```python
from build123d import *

# Parameters (mm, degrees)
F0_W      = 52.5309846
F0_H      = 44.9404867
F0_R      = 1.5
F0_R_2    = 11.2530001
F1_DEPTH  = 5
F2_W      = 3.175
F2_H      = 44.9404867
F3_DEPTH  = 41.774999
F4_W      = 7.9375
F4_H      = 3.175
F5_DEPTH  = 46.774999
F6_R      = 3.96875
F7_R      = 2.2479
F8_DEPTH  = 3.175
F10_DEPTH = 52.5309846
F12_DEPTH = 19.2659
F14_DEPTH = 10.7654979
F15_R     = 7.9375
F16_DEPTH = 25.4
F17_DEPTH = 30.4370867
F18_R     = 3.175
F19_DEPTH = 19.2659
F21_DEPTH = 133
F22_R     = 7.2517
F23_R     = 1.5875


# Not quite as in the source:
# - an extrude ends at something that could not be found from the text; its depth is read off the source's solid
# - a feature names something its author has since deleted; it is built from what else it names


with BuildPart() as f1:
    # F0 (on Top) → F1 (new body)
    with BuildSketch(Plane.XY):
        with Locations((26.2654923, -22.47024335)):
            Rectangle(F0_W, F0_H)
        with Locations((10.7654979, -38.5904867)):
            Circle(F0_R, mode=Mode.SUBTRACT)
        with Locations((26.2654923, -23.0904923)):
            Circle(F0_R_2, mode=Mode.SUBTRACT)
        with Locations((41.7654867, -38.5904867)):
            Circle(F0_R, mode=Mode.SUBTRACT)
        with Locations((10.7654979, -7.5904979)):
            Circle(F0_R, mode=Mode.SUBTRACT)
        with Locations((41.7654867, -7.5904979)):
            Circle(F0_R, mode=Mode.SUBTRACT)
    extrude(amount=F1_DEPTH)

    # F2 (on face) → F3 (join)
    with BuildSketch(Plane(origin=(0, 0, 0), x_dir=(1, 0, 0), z_dir=(0, 0, -1))):
        with Locations((1.5875, 22.47024335)):
            Rectangle(F2_W, F2_H)
        with Locations((50.9434846, 22.47024335)):
            Rectangle(F2_W, F2_H)
    extrude(amount=F3_DEPTH)

    # F4 (on face) → F5 (join, through all)
    with BuildSketch(Plane(origin=(0, 0, -41.774999), x_dir=(1, 0, 0), z_dir=(0, 0, -1))):
        with Locations((-3.96875, 1.5875)):
            Rectangle(F4_W, F4_H)
        with Locations((56.4997346, 1.5875)):
            Rectangle(F4_W, F4_H)
    extrude(amount=-F5_DEPTH)

    # F6
    f6_edges = [f1.edges().sort_by_distance(p)[0] for p in [
        (60.468485, -1.5875, -41.774999),
        (60.468485, -1.5875, 5),
        (-7.9375, -1.5875, 5),
        (-7.9375, -1.5875, -41.774999),
    ]]
    fillet(f6_edges, radius=F6_R)

    # F7 (on face) → F8 (cut, through all)
    with BuildSketch(Plane(origin=(0, 0, 0), x_dir=(-1, 0, 0), z_dir=(0, 1, 0))):
        with Locations((3.96875, -37.806249)):
            Circle(F7_R)
        with Locations((3.96875, 1.03125)):
            Circle(F7_R)
        with Locations((-56.4997346, 1.03125)):
            Circle(F7_R)
        with Locations((-56.4997346, -37.806249)):
            Circle(F7_R)
    extrude(amount=-F8_DEPTH, mode=Mode.SUBTRACT)

    # F9 (on face) → F10 (cut, through all)
    with BuildSketch(Plane.YZ.offset(52.5309846)):
        Polygon((-44.9404867, -3.175), (-44.9404867, -41.774999), (-6.35, -41.774999), align=None)
    extrude(amount=-F10_DEPTH, mode=Mode.SUBTRACT)

    # F11 (on face) → F12 (join)
    with BuildSketch(Plane.XY.offset(5)):
        with BuildLine():
            Line((41.7654867, -44.9404867), (52.5309846, -44.9404867))
            Line((52.5309846, -44.9404867), (52.5309846, -30.4370867))
            Line((52.5309846, -30.4370867), (41.7654867, -30.4370867))
            Line((41.7654867, -30.4370867), (41.7654867, -35.4154867))
            ThreePointArc((41.7654867, -35.4154867), (44.9404867, -38.5904867), (41.7654867, -41.7654867))
            Line((41.7654867, -41.7654867), (41.7654867, -44.9404867))
        make_face()
        with BuildLine():
            Line((52.5309846, -20.7092423), (52.5309846, -12.7717423))
            Line((52.5309846, -12.7717423), (30.7547472146, -12.7717423))
            ThreePointArc((30.7547472146, -12.7717423), (34.966988133, -15.9550889113), (37.2636584966, -20.7092423))
            Line((37.2636584966, -20.7092423), (52.5309846, -20.7092423))
        make_face()
    extrude(amount=F12_DEPTH)

    # F13 (on face) → F14 (cut, through all)
    with BuildSketch(Plane.YZ.offset(52.5309846)):
        with BuildLine():
            Line((-40.0700367, 17.0142), (-37.6887867, 17.0142))
            Line((-37.6887867, 17.0142), (-37.6887867, 14.63295))
            ThreePointArc((-37.6887867, 14.63295), (-36.0049886773, 15.3304019773), (-35.3075367, 17.0142))
            ThreePointArc((-35.3075367, 17.0142), (-37.6887867, 19.39545), (-40.0700367, 17.0142))
        make_face()
        with BuildLine():
            Line((-37.6887867, 14.63295), (-37.6887867, 17.0142))
            Line((-37.6887867, 17.0142), (-40.0700367, 17.0142))
            ThreePointArc((-40.0700367, 17.0142), (-39.3725847227, 15.3304019773), (-37.6887867, 14.63295))
        make_face()
    extrude(amount=-F14_DEPTH, mode=Mode.SUBTRACT)

    # F15 (on face) → F16 (cut)
    with BuildSketch(Plane.XY.offset(5)):
        with Locations((26.2654923, -10.3904923)):
            Circle(F15_R)
    extrude(amount=F16_DEPTH, mode=Mode.SUBTRACT)

    # F17 (add, through all): a face of the model
    f17_faces = [f1.faces().sort_by_distance(p)[0] for p in [
        (47.14823565, -30.4370867, 14.63295),
    ]]
    extrude(f17_faces, amount=F17_DEPTH)

    # F18 (on face) → F19 (cut, through all)
    with BuildSketch(Plane.XY.offset(5)):
        with Locations((41.7654867, -7.5904979)):
            Circle(F18_R)
    extrude(amount=F19_DEPTH, mode=Mode.SUBTRACT)

    # F20 (on face) → F21 (cut, through all)
    with BuildSketch(Plane.YZ.offset(52.5309846)):
        with BuildLine():
            ThreePointArc((-16.7404923, 19.0142), (-18.1547058624, 18.4284135624), (-18.7404923, 17.0142))
            Line((-18.7404923, 17.0142), (-16.7404923, 17.0142))
            Line((-16.7404923, 17.0142), (-16.7404923, 19.0142))
        make_face()
        with BuildLine():
            Line((-16.7404923, 17.0142), (-18.7404923, 17.0142))
            ThreePointArc((-18.7404923, 17.0142), (-16.7404923, 15.0142), (-14.7404923, 17.0142))
            ThreePointArc((-14.7404923, 17.0142), (-15.3262787376, 18.4284135624), (-16.7404923, 19.0142))
            Line((-16.7404923, 19.0142), (-16.7404923, 17.0142))
        make_face()
    extrude(amount=-F21_DEPTH, mode=Mode.SUBTRACT)

    # F22
    f22_edges = [f1.edges().sort_by_distance(p)[0] for p in [
        (47.148236, -44.940487, 24.2659),
    ]]
    fillet(f22_edges, radius=F22_R)

    # F23
    f23_edges = [f1.edges().sort_by_distance(p)[0] for p in [
        (41.765487, -20.709242, 14.63295),
        (41.765487, -12.771742, 14.63295),
    ]]
    fillet(f23_edges, radius=F23_R)


solid = f1.part
```
Part model, mm, in its own coordinate system. A direction names the side the tool comes from. Round coordinates to 2 decimals unless told otherwise and drop trailing zeros. Loops run counter-clockwise (first coordinate to the right, second up) from the corner with the lowest first, then second, coordinate; pieces in that order, holes last. Notation, with made-up numbers: (22, 30.25) -> (72, 30.25) arc R11 cw to (72, 38.25) -> close; hole circle Ø7 at (88.25, -16). An arc over 180 degrees is marked (long way). Use a Markdown table: item, result.
1) Cut at C-C, the plane x = 25.5. List the corners of the cut face in (y, z).
The answers:
| item | result |
|---|---|
| outline | (-44.94, 0) -> (-34.32, 0) -> (-34.32, 5) -> (-44.94, 5) -> close; (-11.86, 0) -> (0, 0) -> (0, 5) -> (-11.86, 5) -> close |
2) Drop flat-ended pins along their axis: pin 1 Ø1.6 at (y, z) = (-44, 17) entering from -X; pin 2 Ø4 at (y, z) = (-38.5, -3) entering from -X; pin 3 Ø13.5 at (y, z) = (-33.5, -10.5) entering from +X. Give the stop position or say it passes through.
The answers:
| item | result |
|---|---|
| pin 1 | stops at x = 41.77 |
| pin 2 | stops at x = 0 |
| pin 3 | stops at x = 52.53 |
3) Cut at A-A, the plane x = 51. State how many separate pieces and enclosed holes the cut face has, and give its area (3 significant figures).
The answers:
| item | result |
|---|---|
| separate pieces | 1 |
| enclosed holes | 2 |
| area | 2,180 mm2 |
4) Cut at B-B, the plane z = -23. List the corners of the cut face in (x, y) (1 decimal).
The answers:
| item | result |
|---|---|
| outline | (-7.9, -3.2) -> (0, -3.2) -> (0, -25.1) -> (3.2, -25.1) -> (3.2, 0) -> (-7.9, 0) -> close; (49.4, -25.1) -> (52.5, -25.1) -> (52.5, -3.2) -> (60.5, -3.2) -> (60.5, 0) -> (49.4, 0) -> close |
5) Tool access for faces 4 (the flat face through (0, -19, -13)), 5 (the flat face through (3.175, -17, -16)), 6 (the flat face through (54, -2, 5)), 7 (the cylindrical face through (41.288, -12.319, 14.768)), 8 (the flat face through (41.765, -29, 14)): list every direction of +Z, -Z, +X, -X, +Y, -Y with a clear straight run to the whole face (end or side of a thin tool).
The answers:
| item | result |
|---|---|
| face 4 | +Z, -Z, -X, -Y |
| face 5 | -Z, +Y, -Y |
| face 6 | +Z, +X, +Y, -Y |
| face 7 | +Z, -X, +Y |
| face 8 | +Z, -X, -Y |
6) Probe line 1 (X direction, y = -8.5, z = -15) (3 decimals); line 2 (Z direction, x = 47, y = -17); line 3 (Z direction, x = 31, y = -40.5). List the from-to ranges inside material, lowest first. Write a range as [from, to].
The answers:
| item | result |
|---|---|
| line 1 | x = [0, 3.175], [49.356, 52.531] |
| line 2 | z = [0, 15.03], [19, 24.27] |
| line 3 | z = [0, 5] |
7) Cut at D-D, the plane y = -28. List the corners of the cut face in (x, z) (3 decimals), and give its area (3 significant figures).
The answers:
| item | result |
|---|---|
| outline | (0, -20.12) -> (3.175, -20.12) -> (3.175, 0) -> (16.14, 0) -> (16.14, 5) -> (0, 5) -> close; (36.391, 0) -> (49.356, 0) -> (49.356, -20.12) -> (52.531, -20.12) -> (52.531, 24.266) -> (41.765, 24.266) -> (41.765, 5) -> (36.391, 5) -> close |
| area | 497 mm2 |
8) Pull direction Y, two halves, no side cores. Call faces 1 (the flat face through (52, -3, -41.775)), 2 (the cylindrical face through (44.94, -7.66, 14.5)), 3 (the flat face through (-4, -3.175, -19)): pulls with the +Y half, pulls with the -Y half, needs draft (parallel to the pull), parting line crosses it, or undercut.
The answers:
| item | result |
|---|---|
| face 1 | needs draft |
| face 2 | undercut |
| face 3 | pulls with the -Y half |
